CAD build for the part. Positions are in the model's coordinates, mm. Round coordinates to 2 decimals unless told otherwise and drop trailing zeros. Order: outer loops, then holes, each group sorted by start corner. A loop starts at its lowest first (then second) coordinate and runs counter-clockwise, first axis right, second up. Notation, with made-up numbers: M 4,79 L 14,79 A34 ccw 14,109 Z; hole C 36,12 d11. An arc over 180 degrees is marked long. Answer as a JSON object with one key per item and string values. Group by question number.
```python
from build123d import *

# Parameters (mm, degrees)
F1_DEPTH = 520


with BuildPart() as f1:
    # F0 (on Top) → F1 (new body)
    with BuildSketch(Plane.XY):
        Polygon((-5, 30.5), (-5, 32), (-10, 32), (-10, -32), (-5, -32), (-5, -30.5), (-8.5, -30.5), (-8.5, -26), (8.5, -26), (8.5, -30.5), (5, -30.5), (5, -32), (10, -32), (10, 32), (5, 32), (5, 30.5), (8.5, 30.5), (8.5, 26), (-8.5, 26), (-8.5, 30.5), align=None)
        Polygon((-8.5, 9.5), (-8.5, 24.5), (8.5, 24.5), (8.5, 9.5), (5.5, 9.5), (5.5, 7.5), (8.5, 7.5), (8.5, -7.5), (5.5, -7.5), (5.5, -9.5), (8.5, -9.5), (8.5, -24.5), (-8.5, -24.5), (-8.5, -9.5), (-5.5, -9.5), (-5.5, -7.5), (-8.5, -7.5), (-8.5, 7.5), (-5.5, 7.5), (-5.5, 9.5), align=None, mode=Mode.SUBTRACT)
    extrude(amount=F1_DEPTH)


solid = f1.part
```
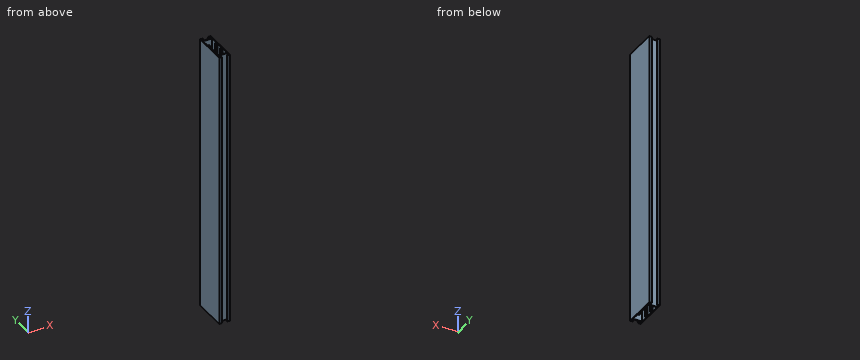
Item 1: Flat gauge pins, fed straight in: pin 1 Ø12 at (x, y) = (-1, 14) entering from +Z; pin 2 Ø1.5 at (x, z) = (-4, 342.5) entering from +Y. Where does each tip first touch, or does it go through?
Item 2: Drill centre lines: line 1 (Y direction, x = -8, z = 283); line 2 (Y direction, x = 2.25, z = 64); line 3 (X direction, y = -21, z = 336). Where is each one in solid material? Low to high. Write a range as [from, to].
Item 3: Cut at B-B, the plane x = 1.25. Give the cut face in (y, z).
Item 4: Cut at A-A, the plane y = 14. Give the cut face in (x, z).
Response values:
{
 "1": {"pin 1": "through", "pin 2": "y = 26"},
 "2": {"line 1": "[-32, -30.5], [-26, -24.5], [-9.5, -7.5], [7.5, 9.5], [24.5, 26], [30.5, 32]", "line 2": "[-26, -24.5], [24.5, 26]", "line 3": "[-10, -8.5], [8.5, 10]"},
 "3": {"outline": "M -26,0 L -24.5,0 L -24.5,520 L -26,520 Z; M 24.5,0 L 26,0 L 26,520 L 24.5,520 Z"},
 "4": {"outline": "M -10,0 L -8.5,0 L -8.5,520 L -10,520 Z; M 8.5,0 L 10,0 L 10,520 L 8.5,520 Z"}
}
